Autodesk Inventor part; units mm, degrees
ref_plane "YZ Plane" through (0, 0, 0) normal (1, 0, 0) x (0, 1, 0)
ref_plane "XZ Plane" through (0, 0, 0) normal (0, 1, 0) x (-1, 0, 0)
ref_plane "XY Plane" through (0, 0, 0) normal (0, 0, 1) x (1, 0, 0)
sketch "Sketch1" plane through (0, 0, 0) normal (0, 0, 1) x (1, 0, 0)
  line L0 (-110.675, 126.35) -> (-171, 126.35)
  line L1 (-171, 126.35) -> (-171, 59.04)
  line L2 (-171, 59.04) -> (-110.675, 59.04)
  line L3 (-110.675, 59.04) -> (-110.675, 126.35)
  point P0 (0, 0)
  dimension "d0" = 60.325
  dimension "d1" = 67.31
extrude "Extrusion1" add sketch "Sketch1" along normal blind 3.175
sketch "Sketch2" plane through (0, 0, 3.175) normal (0, 0, 1) x (1, 0, 0)
  line L0 (-171, 126.35) -> (-171, 59.04)
  line L1 (-171, 59.04) -> (-167.825, 59.04)
  line L2 (-167.825, 59.04) -> (-167.825, 74.915)
  line L3 (-167.825, 74.915) -> (-171, 74.915)
  line L4 (-171, 74.915) -> (-171, 59.04)
  line L5 (-171, 85.075) -> (-167.825, 85.075)
  line L6 (-167.825, 85.075) -> (-167.825, 100.315)
  line L7 (-167.825, 100.315) -> (-171, 100.315)
  line L8 (-171, 100.315) -> (-171, 85.075)
  line L9 (-110.675, 126.35) -> (-171, 126.35)
  line L10 (-171, 126.35) -> (-167.825, 126.35)
  line L11 (-167.825, 126.35) -> (-167.825, 110.475)
  line L12 (-167.825, 110.475) -> (-171, 110.475)
  line L13 (-171, 110.475) -> (-171, 126.35)
  point P0 (0, 0)
  dimension "d4" = 3.175
  dimension "d5" = 15.875
  dimension "d6" = 10.16
  dimension "d7" = 15.875
  dimension "d8" = 10.16
extrude "Extrusion3" cut sketch "Sketch2" against normal blind 3.175
ref_plane "Work Plane1" through (-140.8375, 59.04, 0) normal (1, 0, 0) x (0, 0, -1)
mirror "Mirror1" about plane through (-140.8375, 59.04, 0) normal (1, 0, 0) of "Extrusion3"
sketch "Sketch3" plane through (0, 0, 3.175) normal (0, 0, 1) x (1, 0, 0)
  line L0 (-123.375, 59.04) -> (-110.675, 59.04)
  line L1 (-110.675, 59.04) -> (-110.675, 62.215)
  line L2 (-110.675, 62.215) -> (-123.375, 62.215)
  line L3 (-123.375, 62.215) -> (-123.375, 59.04)
  line L4 (-167.825, 59.04) -> (-113.85, 59.04)
  line L5 (-110.675, 74.915) -> (-110.675, 85.075)
  line L6 (-140.8375, 59.04) -> (-132.265, 59.04)
  line L7 (-132.265, 59.04) -> (-132.265, 62.215)
  line L8 (-132.265, 62.215) -> (-140.8375, 62.215)
  line L9 (-140.8375, 62.215) -> (-140.8375, 59.04)
  point P0 (0, 0)
  dimension "d13" = 12.7
  dimension "d14" = 3.175
  dimension "d15" = 8.89
extrude "Extrusion4" cut sketch "Sketch3" against normal blind 3.175
mirror "Mirror2" about plane through (-140.8375, 59.04, 0) normal (1, 0, 0) of "Extrusion4"
ref_plane "Work Plane2" through (-158.3, 92.695, 0) normal (0, -1, 0) x (1, 0, 0)
mirror "Mirror3" about plane through (-158.3, 92.695, 0) normal (0, -1, 0) of "Extrusion4", "Mirror2"
sketch "Sketch4" plane through (0, 0, 3.175) normal (0, 0, 1) x (1, 0, 0)
  line L0 (-128.1375, 68.565) -> (-153.5375, 68.565)
  line L1 (-153.5375, 68.565) -> (-153.5375, 93.965)
  line L2 (-153.5375, 93.965) -> (-128.1375, 93.965)
  line L3 (-128.1375, 93.965) -> (-128.1375, 68.565)
  line L4 (-149.41, 62.215) -> (-132.265, 62.215)
  line L5 (-140.8375, 151.62) -> (-140.8375, -25.27)
  line L6 (-136.075, 93.965) -> (-145.6, 93.965)
  line L7 (-145.6, 93.965) -> (-145.6, 90.79)
  line L8 (-145.6, 90.79) -> (-136.075, 90.79)
  line L9 (-136.075, 90.79) -> (-136.075, 93.965)
  line L10 (-136.075, 68.565) -> (-145.6, 68.565)
  line L11 (-145.6, 68.565) -> (-145.6, 71.74)
  line L12 (-145.6, 71.74) -> (-136.075, 71.74)
  line L13 (-136.075, 71.74) -> (-136.075, 68.565)
  line L14 (-128.1375, 76.5025) -> (-131.3125, 76.5025)
  line L15 (-131.3125, 76.5025) -> (-131.3125, 86.0275)
  line L16 (-131.3125, 86.0275) -> (-128.1375, 86.0275)
  line L17 (-128.1375, 86.0275) -> (-128.1375, 76.5025)
  line L18 (-153.5375, 76.5025) -> (-150.3625, 76.5025)
  line L19 (-150.3625, 76.5025) -> (-150.3625, 86.0275)
  line L20 (-150.3625, 86.0275) -> (-153.5375, 86.0275)
  line L21 (-153.5375, 86.0275) -> (-153.5375, 76.5025)
  point P0 (0, 0)
  dimension "d18" = 6.35
  dimension "d19" = 12.7
  dimension "d20" = 25.4
  dimension "d21" = 25.4
  dimension "d22" = 7.9375
  dimension "d23" = 7.9375
  dimension "d24" = 3.175
  dimension "d25" = 3.175
  dimension "d26" = 7.9375
  dimension "d27" = 7.9375
  dimension "d28" = 3.175
  dimension "d29" = 3.175
extrude "Extrusion5" cut sketch "Sketch4" against normal blind 3.175 contours L0 L5 L12 L13 | L14 L15 L16 L3 | L0 L11 L12 L5 | L8 L7 L2 L5 | L5 L2 L9 L8 | L1 L20 L19 L18
Build history of the part. All positions in model axes, mm. A direction names the side the tool comes from. Coordinates: 2 decimals unless noted, no trailing zeros. Order: outer loops, then holes, each group sorted by start corner. A loop starts at its lowest first (then second) coordinate and runs counter-clockwise, first axis right, second up. Notation, with made-up numbers: (-2, 8.5) - (8, 8.5) arc R24 cw to (8, 47.5) - close; hole circle Ø4 at (32.5, 26.25). An arc over 180 degrees is marked (long way). Write item = value, one per line. Start each with the question number.
1) Saw through at D-D on z = 0.65. Count the separate pieces of the cut face and the enclosed holes in it, then the cut area to 3 significant figures.
2) Saw through at C-C on y = 78. Write the cut outline in (x, z) (1 decimal), then the cut area to 3 significant figures.
3) Saw through at A-A on y = 70. Write the cut outline in (x, z) (3 decimals).
4) Saw through at B-B on x = -137.5. Write the cut outline in (y, z) (3 decimals).
5) 3-axis set-ups, long thin cutter, end or side, ignore diameter. For faces 5 (the face through (-132.265, 125, 2)), 6 (the face through (-112, 110.475, 2)), 7 (the face through (-152, 76.502, 2)), 8 (the face through (-169, 110.475, 2)): which of +Z, -Z, +X, -X, +Y, -Y reach the whole face in a straight line?
6) Flat gauge pins, fed straight in: pin 1 Ø1 at (x, z) = (-113, 2) entering from -Y (3 decimals); pin 2 Ø1 at (x, z) = (-142, 2) entering from -Y (3 decimals); pin 3 Ø1 at (y, z) = (113.5, 1.5) entering from +X. Where does each tip first touch, or does it go through?
7) Two-plate mould, pull along X, no slides. Class faces 1 (the face through (-113.85, 93, 2)), 2 (the face through (-149.41, 125, 2)), 3 (the face through (-158.3, 61, 2)), 4 (the face through (-163, 62.215, 2)): pulls with the +X half, pulls with the -X half, needs draft (parallel to the pull), parting line crosses it, or undercut.
8) Wall check: line 1 along X through (y, z) = (79.5, 2.05) (1 decimal); line 2 along X through (y, z) = (71, 1.6) (3 decimals); line 3 along Y through (x, z) = (-152, 0.2). Give the ranges that are in metal, low to high. Write a range as from..to.
From the geometry:
q1.separate_pieces = 1
q1.enclosed_holes = 4
q1.area = 3,410 mm^2
q2.outline = (-171, 0) - (-153.5, 0) - (-153.5, 3.2) - (-171, 3.2) - close; (-150.4, 0) - (-131.3, 0) - (-131.3, 3.2) - (-150.4, 3.2) - close; (-128.1, 0) - (-110.7, 0) - (-110.7, 3.2) - (-128.1, 3.2) - close
q2.area = 171 mm^2
q3.outline = (-167.825, 0) - (-145.6, 0) - (-145.6, 3.175) - (-167.825, 3.175) - close; (-136.075, 0) - (-113.85, 0) - (-113.85, 3.175) - (-136.075, 3.175) - close
q4.outline = (62.215, 0) - (68.565, 0) - (68.565, 3.175) - (62.215, 3.175) - close; (71.74, 0) - (90.79, 0) - (90.79, 3.175) - (71.74, 3.175) - close; (93.965, 0) - (123.175, 0) - (123.175, 3.175) - (93.965, 3.175) - close
q5.face_5 = +Z, -Z, +Y
q5.face_6 = +Z, -Z, +X, +Y
q5.face_7 = +Z, -Z
q5.face_8 = +Z, -Z, -X, +Y
q6.pin_1 = 74.915
q6.pin_2 = 62.215
q6.pin_3 = -113.85
q7.face_1 = pulls with the +X half
q7.face_2 = undercut
q7.face_3 = pulls with the -X half
q7.face_4 = needs draft
q8.line_1 = -171..-153.5, -150.4..-131.3, -128.1..-110.7
q8.line_2 = -167.825..-145.6, -136.075..-113.85
q8.line_3 = 59.04..76.5, 86.03..126.35
